Part model, mm, in its own coordinate system. Face numbers are marked on the shaded views. A direction names the side the tool comes from. Give positions to 0.01 mm unless a question says otherwise; leave off trailing zeros. Order: outer loops, then holes, each group sorted by start corner. A loop starts at its lowest first (then second) coordinate and runs counter-clockwise, first axis right, second up. Notation, with made-up numbers: (49.25, -36) - (65.25, -36) arc R30 ccw to (65.25, 3) - close; hole circle Ø8 at (45, 8.25). An arc over 180 degrees is marked (long way). Use one line per item in the form item = value. Start each with the question number.
1. Drill centre lines: line 1 (X direction, y = -5, z = -25.5); line 2 (X direction, y = -3.5, z = -11); line 3 (X direction, y = -2.25, z = -4.5). Where is each one in solid material? Low to high.
2. Pull direction Z, two halves, no side cores. Call the marked faces 4, 5 and 6: +Z half, -Z half, draft (parallel to the pull), parting line (faces both ways), or undercut.
3. Tool access for the marked faces 1, 2 and 3: list every direction of +Z, -Z, +X, -X, +Y, -Y with a clear straight run to the whole face (end or side of a thin tool).
4. Pin check, flat tips, straight feed: P1, Ø6.5, axis at x = 28.5, y = -2, coming from the +Z side (3 decimals); P2, Ø8, axis at x = -9.5, z = -4, coming from the -Y side; P3, Ø2, axis at x = -32.893, y = -3.556, coming from the -Z side; P4, Ø1, axis at y = 3, z = -1, coming from the +X side. Stop position of each tip, or through.
5. Band-saw the part on B-B, the plane x = 6. List the corners of the cut face in (y, z).
6. Band-saw the part on A-A, the plane z = -19.05. State how many separate pieces and enclosed holes the cut face has, plus the area to 3 significant figures.
Autodesk Inventor part; units mm, degrees
ref_plane "Work Plane1" through (-28.321, 6.35, -3.175) normal (-0.2211, 0, -0.9753) x (0, -1, 0)
ref_plane "YZ Plane" through (0, 0, 0) normal (1, 0, 0) x (0, 1, 0)
ref_plane "XZ Plane" through (0, 0, 0) normal (0, 1, 0) x (-1, 0, 0)
sketch "Sketch1" plane through (0, 0, 0) normal (0, 0, 1) x (1, 0, 0)
  line L0 (-50.4952, 0) -> (50.4952, 0)
  line L1 (0, -8.89) -> (0, 8.89)
  line L2 (-36.068, 6.35) -> (36.068, 6.35)
  line L3 (36.068, 6.35) -> (36.068, -6.35)
  line L4 (36.068, -6.35) -> (-36.068, -6.35)
  line L5 (-36.068, -6.35) -> (-36.068, 6.35)
  point P0 (0, 0)
  point P1 (-21.209, 0)
  point P2 (21.209, 0)
  dimension "d0" = 42.418
  dimension "front_mount_width" = 72.136
  dimension "d2" = 12.7
extrude "Extrusion1" add sketch "Sketch1" against normal blind 31.75
sketch "Sketch4" plane through (0, 0, 0) normal (0, 0, 1) x (1, 0, 0)
  line L0 (-50.4952, 0) -> (50.4952, 0)
  line L1 (0, -8.89) -> (0, 8.89)
  line L2 (-36.703, 6.35) -> (-17.653, 6.35)
  line L3 (-17.653, 6.35) -> (-17.653, -6.35)
  line L4 (-17.653, -6.35) -> (-36.703, -6.35)
  line L5 (-36.703, -6.35) -> (-36.703, 6.35)
  line L6 (36.703, 6.35) -> (17.653, 6.35)
  line L7 (17.653, 6.35) -> (17.653, -6.35)
  line L8 (17.653, -6.35) -> (36.703, -6.35)
  line L9 (36.703, -6.35) -> (36.703, 6.35)
  point P0 (0, 0)
  point P1 (-21.209, 0)
  dimension "d8" = 12.7
  dimension "d9" = 19.05
  dimension "d10" = 15.494
sketch "Sketch3" plane through (0, 0, 0) normal (0, 0, 1) x (1, 0, 0)
  line L0 (0, -8.89) -> (0, 8.89)
  line L1 (-50.4952, 0) -> (50.4952, 0)
  point P0 (0, 0)
  point P1 (-21.209, 0)
  point P2 (21.209, 0)
  point P3 (-14.097, 3.556)
  point P4 (-9.525, 3.556)
  point P5 (-14.097, -3.556)
  point P6 (-9.525, -3.556)
  point P7 (14.097, 3.556)
  point P8 (9.525, 3.556)
  point P9 (14.097, -3.556)
  point P10 (9.525, -3.556)
  dimension "d5" = 7.112
  dimension "d6" = 11.684
  dimension "d7" = 3.556
sketch "Sketch6" plane through (-36.068, 6.35, 0) normal (0, 1, 0) x (1, 0, 0)
  line L0 (93.218, 0) -> (-21.082, 0)
  line L1 (-21.082, 0) -> (-21.082, 31.75)
  line L2 (-21.082, 31.75) -> (93.218, 31.75)
  line L3 (93.218, 31.75) -> (93.218, 0)
  line L4 (0, 31.75) -> (72.136, 31.75)
  line L5 (0, 0) -> (72.136, 0)
  line L6 (36.068, 38.1) -> (36.068, -6.35)
  point P0 (36.068, 0)
  dimension "d27" = 57.15
extrude "Extrusion3" [suppressed]
extrude "Extrusion2" cut sketch "Sketch4" against normal blind 3.175
hole "Hole1" [suppressed]
sketch "Sketch5" plane through (0, 0, 0) normal (0, 0, 1) x (1, 0, 0)
  point P0 (0, 0)
  point P1 (-21.209, 0)
  point P2 (21.209, 0)
hole "Hole2" at (-21.209, 0, 0) at (21.209, 0, 0) direction (0, 0, -1) diameter 6.35 depth 50.8 tip angle 118
sketch "Sketch8" plane through (57.15, 9.525, 0) normal (0, 1, 0) x (1, 0, 0)
  line L0 (-57.15, 30.48) -> (-57.15, -5.08)
  line L1 (-114.3, 0) -> (0, 0)
  point P0 (-57.15, 0)
  point P1 (-103.1875, 6.35)
  point P2 (-11.1125, 6.35)
  dimension "d39" = 46.0375
  dimension "d40" = 6.35
hole "Hole4" [suppressed]
sketch "Sketch9" plane through (57.15, 9.525, 0) normal (0, 1, 0) x (1, 0, 0)
  line L0 (-57.15, 30.48) -> (-57.15, -5.08)
  line L1 (-114.3, 0) -> (0, 0)
  point P0 (-57.15, 0)
  point P1 (-86.3092, 6.35)
  point P2 (-27.9908, 6.35)
  dimension "d48" = 58.3184
  dimension "d49" = 6.35
hole "Hole5" [suppressed]
sketch "Sketch10" plane through (-36.068, 6.35, 0) normal (0, 1, 0) x (1, 0, 0)
  line L0 (6.9088, 25.4) -> (6.9088, 8.89) construction
  line L1 (4.4196, 25.4) -> (4.4196, 8.89)
  line L2 (9.398, 8.89) -> (9.398, 25.4)
  arc A0 (9.398, 25.4) -> (4.4196, 25.4) centre (6.9088, 25.4) ccw
  arc A1 (4.4196, 8.89) -> (9.398, 8.89) centre (6.9088, 8.89) ccw
  line L3 (36.068, 38.1) -> (36.068, -6.35)
  line L4 (67.7164, 25.4) -> (67.7164, 8.89)
  line L5 (62.738, 8.89) -> (62.738, 25.4)
  arc A2 (67.7164, 25.4) -> (62.738, 25.4) centre (65.2272, 25.4) ccw
  arc A3 (62.738, 8.89) -> (67.7164, 8.89) centre (65.2272, 8.89) ccw
  line L6 (0, 0) -> (72.136, 0)
  line L7 (0, 31.75) -> (72.136, 31.75)
  point P0 (36.068, 0)
  point P1 (6.9088, 17.145)
  dimension "d57" = 58.3184
  dimension "d58" = 4.9784
  dimension "d59" = 8.89
  dimension "d60" = 6.35
extrude "Extrusion4" [suppressed]
sketch "Sketch12" plane through (0, 0, 0) normal (0, 0, 1) x (1, 0, 0)
  line L0 (-50.4952, 0) -> (50.4952, 0)
  line L1 (0, -8.89) -> (0, 8.89)
  point P0 (0, 0)
  point P1 (-21.209, 0)
  point P2 (-28.321, 3.556)
  point P3 (-32.893, 3.556)
  point P4 (-28.321, -3.556)
  point P5 (-32.893, -3.556)
  point P6 (28.321, 3.556)
  point P7 (32.893, 3.556)
  point P8 (32.893, -3.556)
  point P9 (28.321, -3.556)
  dimension "d63" = 7.112
  dimension "d64" = 11.684
  dimension "d65" = 3.556
hole "Hole6" at (-32.893, 3.556, 0) at (-28.321, 3.556, 0) at (-32.893, -3.556, 0) at (-28.321, -3.556, 0) at (28.321, 3.556, 0) at (32.893, 3.556, 0) at (28.321, -3.556, 0) at (32.893, -3.556, 0) direction (0, 0, -1) diameter 1.7018 depth 50.8 tip angle 118
sketch "Sketch13" plane through (-36.068, -6.35, -31.75) normal (0, -1, 0) x (1, 0, 0)
  line L0 (36.068, -6.35) -> (36.068, 38.1)
  line L1 (-14.4272, 31.75) -> (86.5632, 31.75)
  line L2 (53.721, 31.75) -> (18.415, 31.75)
  line L3 (21.7805, 31.75) -> (50.3555, 31.75)
  line L4 (50.3555, 31.75) -> (50.3555, 0)
  line L5 (50.3555, 0) -> (21.7805, 0)
  line L6 (21.7805, 0) -> (21.7805, 31.75)
  line L7 (72.136, 0) -> (0, 0)
  point P0 (36.068, 31.75)
  point P1 (36.068, 0)
  point P2 (20.712, 10.7844)
  dimension "d73" = 28.575
extrude "Extrusion5" cut sketch "Sketch13" against normal blind 6.35
chamfer "Chamfer1" [suppressed]
sketch "Sketch14" plane through (-36.068, 6.35, -31.75) normal (0, 1, 0) x (1, 0, 0)
  line L0 (36.068, 6.35) -> (36.068, -38.1)
  line L1 (18.415, -31.75) -> (53.721, -31.75)
  point P0 (36.068, -31.75)
  point P1 (6.8724, -6.35)
  point P2 (65.2636, -6.35)
  dimension "d79" = 25.4
hole "Hole7" at (-29.1956, 6.35, -25.4) at (29.1956, 6.35, -25.4) direction (0, -1, 0) diameter 4.9784 depth 25.4 tip angle 118
sketch "Sketch15" plane through (-36.068, 6.35, -31.75) normal (0, 1, 0) x (1, 0, 0)
  line L0 (36.068, 6.35) -> (36.068, -38.1) construction
  line L1 (18.415, -31.75) -> (53.721, -31.75)
  point P0 (36.068, -31.75)
  point P1 (26.543, -12.7)
  point P2 (45.593, -12.7)
  dimension "d87" = 19.05
  dimension "d88" = 9.525
hole "Hole8" at (-9.525, 6.35, -19.05) at (9.525, 6.35, -19.05) direction (0, -1, 0) diameter 4.9784 depth 14.9352 tip angle 118
sketch "Sketch16" plane through (0, 0, 0) normal (0, 0, 1) x (1, 0, 0)
  line L0 (-14.2875, 0) -> (14.2875, 0)
  line L1 (0, -8.89) -> (0, 8.89)
  point P0 (0, 0)
  point P1 (0, 0)
  point P2 (0, 2.349)
  dimension "d96" = 2.349
hole "Hole9" [suppressed]
sketch "Sketch17" plane through (0, 0, -3.175) normal (0, 0, 1) x (1, 0, 0)
  point P0 (0, 0)
  point P1 (-21.209, 0)
  point P2 (21.209, 0)
hole "Hole10" [suppressed]
sketch "Sketch18" plane through (-36.068, 6.35, -31.75) normal (0, 1, 0) x (1, 0, 0)
  line L0 (8.5979, -28.575) -> (6.8961, -28.575)
  line L1 (6.8961, 0) -> (8.5979, 0)
  line L2 (0, 0) -> (7.747, -28.575) construction
  line L3 (0, 0) -> (6.8961, 0) construction
  line L4 (7.747, -28.575) -> (1.27, 0)
  line L5 (7.0959, -28.575) -> (0.6189, 0) construction
  line L6 (-2.0115, -15.6677) -> (-0.7269, -12.645) construction
  line L7 (8.3345, -28.2943) -> (1.8575, 0.2807) construction
  point P0 (36.068, -31.75)
  dimension "d111" = 1.27
  dimension "d112" = 0.635
ref_plane "Work Plane1" through (-28.321, 6.35, -3.175) normal (-0.2211, 0, -0.9753) x (0, -1, 0)
sketch "Sketch19" plane through (-28.321, 6.35, -3.175) normal (-0.2211, 0, -0.9753) x (0, -1, 0)
  line L0 (6.35, 22.3275) -> (6.35, -76.1645)
  line L1 (0, 0) -> (6.35, 0) construction
  point P0 (6.35, -26.9185)
hole "Hole11" at (-28.321, 0, -3.175) direction (-0.2211, 0, -0.9753) diameter 2.032 end through all both
chamfer "Chamfer2" distance 0.762 angle 45 1 edges at (-28.321, 1.016, -3.175)
sketch "Sketch20" plane through (0, 0, 0) normal (0, 0, 1) x (1, 0, 0)
  line L0 (-14.2875, -6.35) -> (-36.068, -6.35)
  line L1 (-14.2875, -6.35) -> (-17.653, -6.35)
  line L2 (-17.653, -6.35) -> (-17.653, 6.35)
  line L3 (-17.653, 6.35) -> (-14.2875, 6.35)
  line L4 (-14.2875, 6.35) -> (-14.2875, -6.35)
  line L5 (14.2875, -6.35) -> (14.2875, 0)
  line L6 (17.653, 6.35) -> (36.068, 6.35)
  line L7 (14.2875, -6.35) -> (17.653, -6.35)
  line L8 (17.653, -6.35) -> (17.653, 6.35)
  line L9 (17.653, 6.35) -> (14.2875, 6.35)
  line L10 (14.2875, 6.35) -> (14.2875, -6.35)
  point P0 (0, 0)
extrude "Extrusion6" [suppressed]
sketch "Sketch21" plane through (0, 0, 0) normal (0, 0, 1) x (1, 0, 0)
  line L0 (-17.653, 6.35) -> (-17.653, -6.35)
  line L1 (17.653, -6.35) -> (17.653, 6.35)
  line L2 (-17.653, -6.35) -> (17.653, -6.35)
  line L3 (17.653, -6.35) -> (17.653, 0)
  line L4 (17.653, 0) -> (-17.653, 0)
  line L5 (-17.653, 0) -> (-17.653, -6.35)
  point P0 (0, 0)
extrude "Extrusion7" cut sketch "Sketch21" against normal blind 50.8
sketch "Sketch22" plane through (0, 0, 0) normal (0, 0, 1) x (1, 0, 0)
  point P0 (0, 0)
properties part number "v2_front_ mount_2" material "Aluminum 6061"
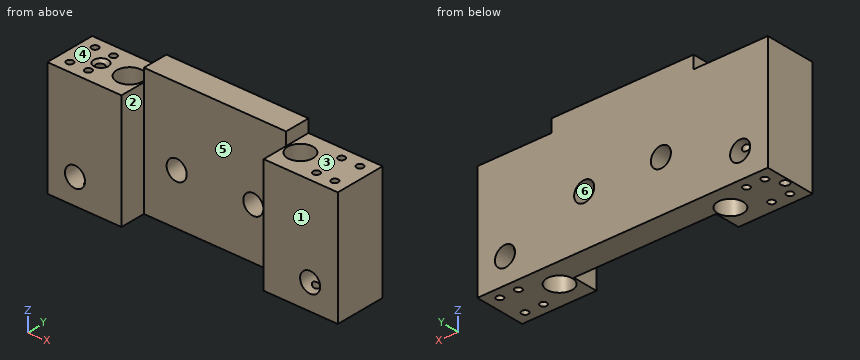
From the geometry:
q1.line_1 = -36.07 to -31.68, -26.71 to -17.65, 17.65 to 26.71, 31.68 to 36.07
q1.line_2 = -36.07 to -33.74, -32.04 to -29.17, -27.47 to -17.65, 17.65 to 27.47, 29.17 to 32.04, 33.74 to 36.07
q1.line_3 = -36.07 to -23.45, -18.97 to -17.65, 17.65 to 18.97, 23.45 to 36.07
q2.face_4 = +Z half
q2.face_5 = draft
q2.face_6 = undercut
q3.face_1 = +Z, -Z, +X, -X, -Y
q3.face_2 = +Z, -Z, -Y
q3.face_3 = +Z, +X, +Y, -Y
q4.P1 = -3.175
q4.P2 = 0
q4.P3 = -31.75
q4.P4 = 17.65
q5.outline = (0, -31.75) - (6.35, -31.75) - (6.35, 0) - (0, 0) - close
q6.separate_pieces = 3
q6.enclosed_holes = 11
q6.area = 544 mm²
